```python
from build123d import *

# Parameters (mm, degrees)
SKETCH1_W           = 266.7
SKETCH1_H           = 127
BOSS_EXTRUDE1_DEPTH = 19.05
SKETCH2_W           = 19.05
SKETCH2_H           = 76.2
CUT_EXTRUDE1_DEPTH  = 149.920700374
SKETCH3_W           = 25.4
SKETCH3_H           = 6.35
BOSS_EXTRUDE2_DEPTH = 25.4
SKETCH5_W           = 6.35
SKETCH5_H           = 6.35
CUT_EXTRUDE2_DEPTH  = 190.438710405
SKETCH6_W           = 1.27
SKETCH6_H           = 5.08
CUT_EXTRUDE3_DEPTH  = 190.438710405
SKETCH7_W           = 0.254
SKETCH7_H           = 12.446
SKETCH7_W_2         = 4.318
SKETCH7_H_2         = 0.254
CUT_EXTRUDE4_DEPTH  = 190.438710405
SKETCH8_W           = 50.8
SKETCH8_H           = 6.35
BOSS_EXTRUDE3_DEPTH = 12.7
CUT_EXTRUDE5_REACH  = 157.575
SKETCH9_W           = 44.45
SKETCH9_H           = 6.35


with BuildPart() as part:
    # Sketch1 → Boss-Extrude1 (new body)
    with BuildSketch(Plane(origin=(0, 0, 0), x_dir=(1, 0, 0), z_dir=(0, 1, 0))):
        Rectangle(SKETCH1_W, SKETCH1_H)
    extrude(amount=BOSS_EXTRUDE1_DEPTH)

    # Sketch2 → Cut-Extrude1 (cut, through all)
    with BuildSketch(Plane(origin=(0, 19.05, 0), x_dir=(1, 0, 0), z_dir=(0, 1, 0))):
        with Locations((-123.825, 0)):
            Rectangle(SKETCH2_W, SKETCH2_H)
    cut_extrude1 = extrude(amount=-CUT_EXTRUDE1_DEPTH, mode=Mode.SUBTRACT)

    # Mirror1: Cut-Extrude1 across plane
    add(cut_extrude1.mirror(Plane(origin=(0, 0, 0), x_dir=(0, 0, 1), z_dir=(1, 0, 0))), mode=Mode.SUBTRACT)

    # Sketch3 → Boss-Extrude2 (add)
    with BuildSketch(Plane(origin=(0, 19.05, 0), x_dir=(1, 0, 0), z_dir=(0, 1, 0))):
        with Locations((0, -60.325)):
            Rectangle(SKETCH3_W, SKETCH3_H)
    boss_extrude2 = extrude(amount=BOSS_EXTRUDE2_DEPTH)

    # Sketch5 → Cut-Extrude2 (cut, through all)
    with BuildSketch(Plane.XY.offset(63.5)):
        with Locations((3.175, 41.275)):
            Rectangle(SKETCH5_W, SKETCH5_H)
    cut_extrude2 = extrude(amount=-CUT_EXTRUDE2_DEPTH, mode=Mode.SUBTRACT)

    # Sketch6 → Cut-Extrude3 (cut, through all)
    with BuildSketch(Plane.XY.offset(63.5)):
        with Locations((6.985, 40.64)):
            Rectangle(SKETCH6_W, SKETCH6_H)
    cut_extrude3 = extrude(amount=-CUT_EXTRUDE3_DEPTH, mode=Mode.SUBTRACT)

    # Sketch7 → Cut-Extrude4 (cut, through all)
    with BuildSketch(Plane.XY.offset(63.5)):
        with Locations((7.493, 31.877)):
            Rectangle(SKETCH7_W, SKETCH7_H)
        with Locations((9.779, 25.527)):
            Rectangle(SKETCH7_W_2, SKETCH7_H_2)
        with Locations((7.493, 25.527)):
            Rectangle(SKETCH7_W, SKETCH7_H_2)
    cut_extrude4 = extrude(amount=-CUT_EXTRUDE4_DEPTH, mode=Mode.SUBTRACT)

    # Mirror2: Boss-Extrude2, Cut-Extrude2, Cut-Extrude3, Cut-Extrude4 across plane
    add(boss_extrude2.mirror(Plane.XY))
    add(cut_extrude2.mirror(Plane.XY), mode=Mode.SUBTRACT)
    add(cut_extrude3.mirror(Plane.XY), mode=Mode.SUBTRACT)
    add(cut_extrude4.mirror(Plane.XY), mode=Mode.SUBTRACT)

    # Sketch8 → Boss-Extrude3 (add)
    with BuildSketch(Plane(origin=(0, 19.05, 0), x_dir=(1, 0, 0), z_dir=(0, 1, 0))):
        Rectangle(SKETCH8_W, SKETCH8_H)
    extrude(amount=BOSS_EXTRUDE3_DEPTH)

    # Sketch9 → Cut-Extrude5 (cut, up to next)
    with BuildSketch(Plane.XY.offset(3.175), mode=Mode.PRIVATE) as cut_extrude5_sk1:
        with Locations((0, 31.75)):
            Rectangle(SKETCH9_W, SKETCH9_H)
    cut_extrude5_tool1 = extrude(cut_extrude5_sk1.sketch, amount=-CUT_EXTRUDE5_REACH, mode=Mode.PRIVATE) & part.part
    add(cut_extrude5_tool1.solids().sort_by_distance((0, 31.75, 3.175))[0], mode=Mode.SUBTRACT)


solid = part.part
```
Could you check a few things on this model? Use its own coordinates, in mm. A direction names the side the tool comes from. Coordinates: 2 decimals unless noted, no trailing zeros. Order: outer loops, then holes, each group sorted by start corner. A loop starts at its lowest first (then second) coordinate and runs counter-clockwise, first axis right, second up. Notation, with made-up numbers: M 81.5,-19.75 L 94.5,-19.75 A18 cw 94.5,-1.75 Z; hole C 83.5,-17 d9. An arc over 180 degrees is marked long. Use one line per item in the form item = value. Start each with the question number.
1. Suppose I cut it at A-A on y = 40.5. Write out the boundary of the cut face in (x, z).
2. Suppose I cut it at D-D on y = 8.5. Write out the boundary of the cut face in (x, z), then the cut area to 3 significant figures.
3. Suppose I cut it at B-B on x = -7.5. Write out the boundary of the cut face in (y, z) (3 decimals).
4. On a 3-axis mill with a long thin cutter (end or side, diameter ignored), from which of +Z, -Z, +X, -X, +Y, -Y can I reach the whole of each face in a straight line? I mean faces 1 (the flat face through (-114.3, 10, 1)), 2 (the flat face through (12.7, 32, -60)), 3 (the flat face through (0, 24, -3.175)), 4 (the flat face through (10, 25.4, -60)), 5 (the flat face through (12.7, 32, 60)). Say none if no direction works.
5. We'd pull the mould along X, two halves only. Please class faces 6 (the flat face through (0, 28.575, 0)), 7 (the flat face through (-12.7, 32, -60)), 8 (the flat face through (-6, 44.45, -60)), 9 (the flat face through (7.62, 34, 60)): +X half, -X half, draft (parallel to the pull), parting line (faces both ways), or undercut.
6. For pin 1 (3 mm diameter, centred on y = 38, z = -62, fed in from -X); pin 2 (21 mm diameter, centred on y = 13, z = -17, fed in from +X); pin 3 (1.9 mm diameter, centred on x = 1, z = -0.5, fed in from +Y) (3 decimals), each with a flat end and sliding along its axis, tell me the tip position at first contact or that it passes through.
7. Suppose I cut it at C-C on z = 40.5. Write out the boundary of the cut face in (x, y).
8. Please list where these lines run through material, in increasing order: line 1 (Z direction, x = 115, y = 15.5); line 2 (Y direction, x = 21, z = 22); line 3 (X direction, y = 7.5, z = 24).
Geometry says:
q1.outline = M -12.7,-63.5 L 0,-63.5 L 0,-57.15 L -12.7,-57.15 Z; M -12.7,57.15 L 0,57.15 L 0,63.5 L -12.7,63.5 Z; M 7.62,-63.5 L 12.7,-63.5 L 12.7,-57.15 L 7.62,-57.15 Z; M 7.62,57.15 L 12.7,57.15 L 12.7,63.5 L 7.62,63.5 Z
q2.outline = M -133.35,-63.5 L 133.35,-63.5 L 133.35,-38.1 L 114.3,-38.1 L 114.3,38.1 L 133.35,38.1 L 133.35,63.5 L -133.35,63.5 L -133.35,38.1 L -114.3,38.1 L -114.3,-38.1 L -133.35,-38.1 Z
q2.area = 31,000 mm^2
q3.outline = M 0,-63.5 L 44.45,-63.5 L 44.45,-57.15 L 19.05,-57.15 L 19.05,-3.175 L 28.575,-3.175 L 28.575,3.175 L 19.05,3.175 L 19.05,57.15 L 44.45,57.15 L 44.45,63.5 L 0,63.5 Z
q4.face_1 = -X, +Y, -Y
q4.face_2 = -Z, +X, +Y
q4.face_3 = +X, -X, +Y
q4.face_4 = -Z
q4.face_5 = +Z, +X, +Y
q5.face_6 = undercut
q5.face_7 = -X half
q5.face_8 = draft
q5.face_9 = undercut
q6.pin_1 = -12.7
q6.pin_2 = 114.3
q6.pin_3 = 28.575
q7.outline = M -133.35,0 L 133.35,0 L 133.35,19.05 L -133.35,19.05 Z
q8.line_1 = -63.5 to -38.1, 38.1 to 63.5
q8.line_2 = 0 to 19.05
q8.line_3 = -114.3 to 114.3
